The drawing under review shows one solid part. Ordinate dimensions are in mm from its lowest x, y, z. Round coordinates to 2 decimals unless told otherwise and drop trailing zeros. Order: outer loops, then holes, each group sorted by start corner. A loop starts at its lowest first (then second) coordinate and runs counter-clockwise, first axis right, second up. Notation, with made-up numbers: (-25.75, 71.25) -> (-13.75, 71.25) arc R27 cw to (-13.75, 96.25) -> close; hole circle Ø3 at (88, 48). An arc over 180 degrees is marked (long way). Use a Markdown table: item, result. Add a question column.
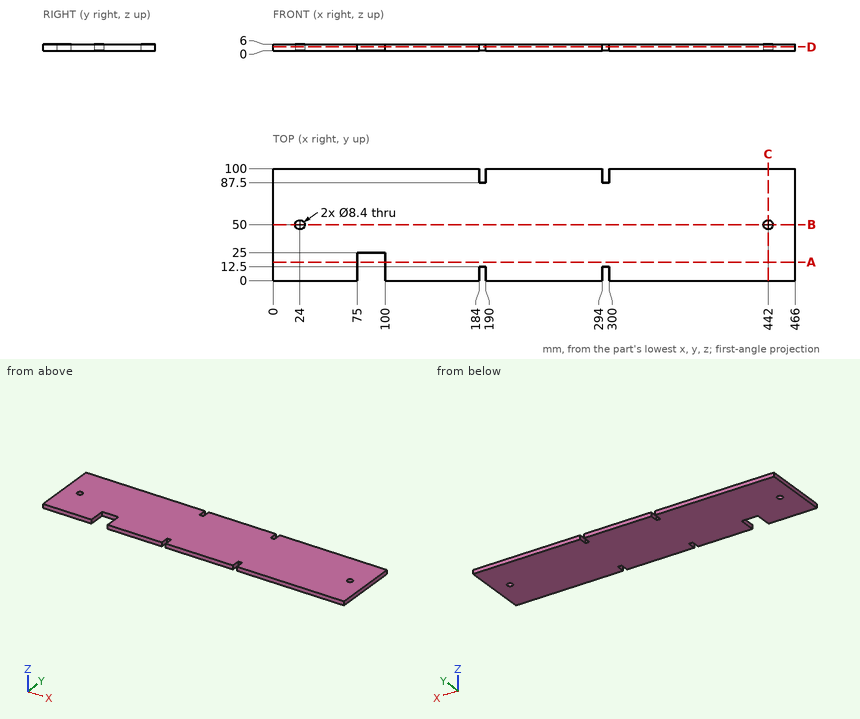
Q1. Add section D-D, the plane z = 3.35. Give the boundary of the cut face in (x, y), then the cut area to 3 significant figures.
Q2. For pin 1 (3 mm diameter, centred on y = 8, z = 1.5, fed in from -X); pin 2 (3 mm diameter, centred on x = 296.5, z = 3, fed in from -Y); pin 3 (1 mm diameter, centred on x = 77, z = 1.5, fed in from -Y); pin 4 (5 mm diameter, centred on x = 24, y = 50, fed in from -Z), all flat-tipped, find the tip position at first contact; note any pin that passes through.
Q3. Add section C-C, the plane x = 442. Give the boundary of the cut face in (y, z), then the cut area to 3 significant figures.
Q4. To check wall thickness, follow line 1 along X through (y, z) = (90, 0.2); line 2 along Y through (x, z) = (442, 3.2); line 3 along X through (y, z) = (48, 0.9). State the ranges of each line that lie inside material, in increasing order.
Q5. Add section B-B, the plane y = 50. Give the boundary of the cut face in (x, z), then the cut area to 3 significant figures.
Q6. Add section A-A, the plane y = 16.5. Give the boundary of the cut face in (x, z).
Return value:
| question | item | result |
|---|---|---|
| 1 | outline | (0, 0) -> (75, 0) -> (75, 25) -> (100, 25) -> (100, 0) -> (184, 0) -> (184, 12.5) -> (190, 12.5) -> (190, 0) -> (294, 0) -> (294, 12.5) -> (300, 12.5) -> (300, 0) -> (466, 0) -> (466, 100) -> (300, 100) -> (300, 87.5) -> (294, 87.5) -> (294, 100) -> (190, 100) -> (190, 87.5) -> (184, 87.5) -> (184, 100) -> (0, 100) -> close; hole circle Ø8.4 at (24, 50); hole circle Ø8.4 at (442, 50) |
| 1 | area | 45,600 mm² |
| 2 | pin 1 | x = 0 |
| 2 | pin 2 | y = 12.5 |
| 2 | pin 3 | y = 25 |
| 2 | pin 4 | through |
| 3 | outline | (0, 0) -> (45.8, 0) -> (45.8, 6) -> (0, 6) -> close; (54.2, 0) -> (100, 0) -> (100, 6) -> (54.2, 6) -> close |
| 3 | area | 550 mm² |
| 4 | line 1 | 0 to 184, 190 to 294, 300 to 466 |
| 4 | line 2 | 0 to 45.8, 54.2 to 100 |
| 4 | line 3 | 0 to 20.31, 27.69 to 438.31, 445.69 to 466 |
| 5 | outline | (0, 0) -> (19.8, 0) -> (19.8, 6) -> (0, 6) -> close; (28.2, 0) -> (437.8, 0) -> (437.8, 6) -> (28.2, 6) -> close; (446.2, 0) -> (466, 0) -> (466, 6) -> (446.2, 6) -> close |
| 5 | area | 2,700 mm² |
| 6 | outline | (0, 0) -> (75, 0) -> (75, 6) -> (0, 6) -> close; (100, 0) -> (466, 0) -> (466, 6) -> (100, 6) -> close |
